from build123d import *

# Parameters (mm, degrees)
F1_W     = 116
F1_H     = 116
F1_R     = 51.5
F1_R_2   = 48.75
F2_DEPTH = 6
F3_DEPTH = 30
F4_DEPTH = 6
F5_DEPTH = 6


with BuildPart() as f2:
    # F1 (on Top) → F2 (new body)
    with BuildSketch(Plane.XY):
        Rectangle(F1_W, F1_H)
        Circle(F1_R, mode=Mode.SUBTRACT)
        Circle(F1_R)
        Circle(F1_R_2, mode=Mode.SUBTRACT)
    extrude(amount=-F2_DEPTH)

    # F1 (on Top) → F3 (join)
    with BuildSketch(Plane.XY):
        Circle(F1_R)
        Circle(F1_R_2, mode=Mode.SUBTRACT)
    extrude(amount=F3_DEPTH)

    # F0 (on Top) → F4 (cut)
    with BuildSketch(Plane.XY):
        with BuildLine():
            Line((16, 53.5), (19, 53.5))
            ThreePointArc((19, 53.5), (17.5, 55), (16, 53.5))
        make_face()
        with BuildLine():
            ThreePointArc((16, 53.5), (17.5, 52), (19, 53.5))
            Line((19, 53.5), (16, 53.5))
        make_face()
    extrude(amount=-F4_DEPTH, mode=Mode.SUBTRACT)

    # F0 (on Top) → F5 (cut)
    with BuildSketch(Plane.XY):
        with BuildLine():
            Line((16, -53.5), (19, -53.5))
            ThreePointArc((19, -53.5), (17.5, -52), (16, -53.5))
        make_face()
        with BuildLine():
            ThreePointArc((16, -53.5), (17.5, -55), (19, -53.5))
            Line((19, -53.5), (16, -53.5))
        make_face()
        with BuildLine():
            Line((-19, -53.5), (-16, -53.5))
            ThreePointArc((-16, -53.5), (-17.5, -52), (-19, -53.5))
        make_face()
        with BuildLine():
            ThreePointArc((-19, -53.5), (-17.5, -55), (-16, -53.5))
            Line((-16, -53.5), (-19, -53.5))
        make_face()
        with BuildLine():
            ThreePointArc((-19, 53.5), (-17.5, 52), (-16, 53.5))
            Line((-16, 53.5), (-19, 53.5))
        make_face()
        with BuildLine():
            Line((-19, 53.5), (-16, 53.5))
            ThreePointArc((-16, 53.5), (-17.5, 55), (-19, 53.5))
        make_face()
    extrude(amount=-F5_DEPTH, mode=Mode.SUBTRACT)


with BuildPart() as f2_1:
    # F6: moved
    add(f2.part.moved(Location((0, 0, 6))))


solid = f2_1.part
Input: part model. Units: mm. Frame: model coordinates. A direction names the side the tool comes from. Give positions to 0.01 mm unless a question says otherwise; leave off trailing zeros. Write each loop counter-clockwise with the first axis right and the second up, starting at its lowest first coordinate (ties: lowest second). Pieces come first, ordered by that corner, then holes. Notation, with made-up numbers: M 27.5,20 L 82.5,20 A29 ccw 82.5,40 Z; hole C -2,81 d7. An arc over 180 degrees is marked long. Write item = value, one per line. Start each with the question number.
1) Reachability of faces 1 (the cylindrical face through (18.7, -52.6, 3)), 2 (the flat face through (-52, 1, 6)) from +Z, -Z, +X, -X, +Y, -Y: full face, straight path, thin tool, end or side. Return the list, or none.
2) Cut plane B-B on y = -53.5. Return the cut outline in (x, z).
3) Material intervals for line 1 along X through (y, z) = (-53.5, 1.9); line 2 along Y through (x, z) = (-17, 4); line 3 along X through (y, z) = (-53, 4), sorted ascending. Write a range as [from, to].
4) Cut plane D-D on x = 17.5. Return the cut outline in (y, z), then the cut area to 3 significant figures.
5) First-contact query: pin 1 Ø1.5 at (x, z) = (-41.5, 29.5) entering from +Y; pin 2 Ø4 at (x, z) = (-22.5, 18.5) entering from -Y; pin 3 Ø10 at (y, z) = (-27.5, 19) entering from -X. Flat tips, straight axial feed; report the tip coordinate or a pass-through.
6) Draft query along X for faces 3 (the flat face through (-31, -38, 36)), 4 (the cylindrical face through (-11.164, -50.275, 20.79)), 5 (the cylindrical face through (-38.69, -29.66, 17.75)). Return one class per face: +X half, -X half, draft (parallel to the pull), parting line (faces both ways), or undercut.
7) Cut plane A-A on x = 0. Return the cut outline in (y, z).
Solved:
q1.face_1 = +Z, -Z
q1.face_2 = +Z
q2.outline = M -58,0 L -19,0 L -19,6 L -58,6 Z; M -16,0 L 16,0 L 16,6 L -16,6 Z; M 19,0 L 58,0 L 58,6 L 19,6 Z
q3.line_1 = [-58, -19], [-16, 16], [19, 58]
q3.line_2 = [-58, -54.91], [-52.09, -45.69], [45.69, 52.09], [54.91, 58]
q3.line_3 = [-58, -18.91], [-16.09, 16.09], [18.91, 58]
q4.outline = M -58,0 L -55,0 L -55,6 L -58,6 Z; M -52,0 L -45.5,0 L -45.5,36 L -48.44,36 L -48.44,6 L -52,6 Z; M 45.5,0 L 52,0 L 52,6 L 48.44,6 L 48.44,36 L 45.5,36 Z; M 55,0 L 58,0 L 58,6 L 55,6 Z
q4.area = 290 mm2
q5.pin_1 = 31.49
q5.pin_2 = -47.24
q5.pin_3 = -46.32
q6.face_3 = draft
q6.face_4 = parting line
q6.face_5 = undercut
q7.outline = M -58,0 L -48.75,0 L -48.75,36 L -51.5,36 L -51.5,6 L -58,6 Z; M 48.75,0 L 58,0 L 58,6 L 51.5,6 L 51.5,36 L 48.75,36 Z
